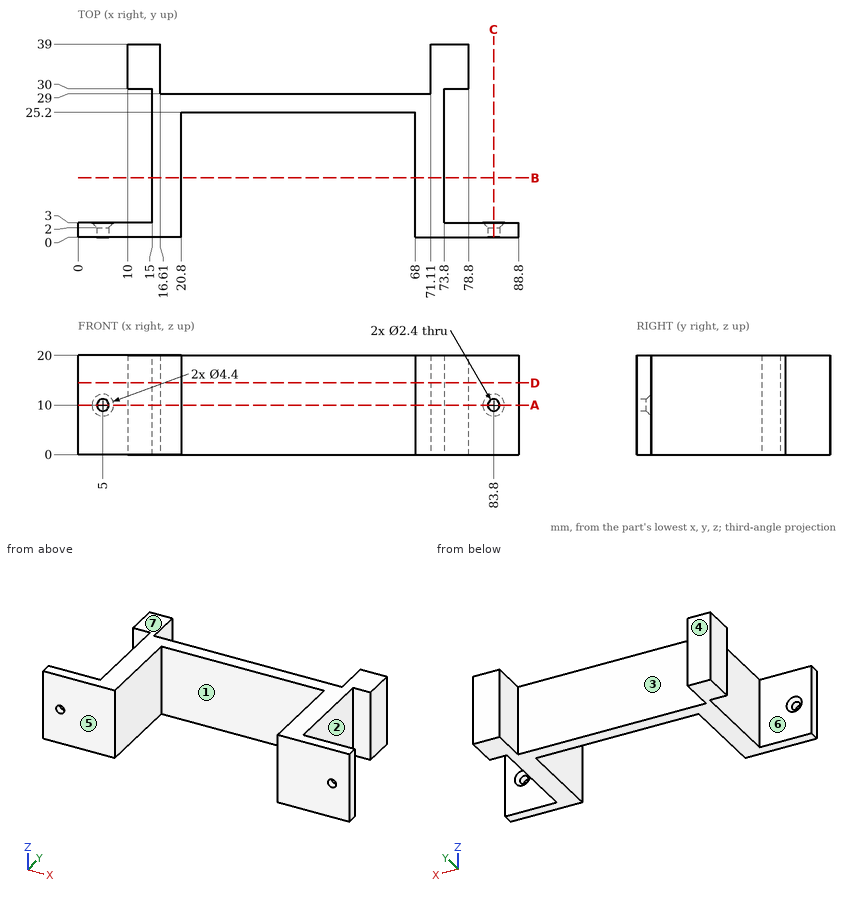
Design review of the part shown in the three views and the two pictorial views. Dimensions are in mm from the part's minimum x, y and z. A direction names the side the tool comes from. Give positions to 0.01 mm unless a question says otherwise; leave off trailing zeros. Write each loop counter-clockwise with the first axis right and the second up, starting at its lowest first coordinate (ties: lowest second). Pieces come first, ordered by that corner, then holes. Notation, with made-up numbers: M 36,45.25 L 76,45.25 A8 ccw 76,55.25 Z; hole C 39,12 d7. An arc over 180 degrees is marked long. Answer as CSV lines item,"result".
1. Draft analysis for pull direction Y (two halves, no side actions). For the marked faces 4, 5, 6 and 7, state which applies: +Y half, -Y half, draft (parallel to the pull), parting line (faces both ways), or undercut.
Findings:
face 4,"+Y half"
face 5,"-Y half"
face 6,"undercut"
face 7,"draft"
2. For the marked faces 1, 2 and 3, list the 3-axis set-ups (+Z, -Z, +X, -X, +Y, -Y) from which the entire face can be reached by the end or side of a thin tool; tool diameter is ignored.
Findings:
face 1,"+Z, -Z, -Y"
face 2,"+Z, -Z, +X"
face 3,"+Z, -Z, +Y"
3. Consider section B-B, the plane y = 12. Write out the cut boundary in (x, z), then the cut area to 3 significant figures.
Findings:
outline,"M 15,0 L 20.8,0 L 20.8,20 L 15,20 Z; M 68,0 L 73.8,0 L 73.8,20 L 68,20 Z"
area,"232 mm2"
4. Consider section C-C, the plane x = 83.8. Write out the cut boundary in (y, z), then the cut area to 3 significant figures.
Findings:
outline,"M 0,0 L 3,0 L 3,7.8 L 2,8.8 L 0,8.8 Z; M 0,11.2 L 2,11.2 L 3,12.2 L 3,20 L 0,20 Z"
area,"51.8 mm2"
5. Wall thickness on line 1 (X direction, y = 1.15, z = 10); line 2 (X direction, y = 15, z = 4.5); line 3 (Z direction, x = 5, y = 1.25): over which ranges is each line inside the solid? List them lowest first.
Findings:
line 1,"x = 0 to 3.8, 6.2 to 20.8, 68 to 82.6, 85 to 88.8"
line 2,"x = 15 to 20.8, 68 to 73.8"
line 3,"z = 0 to 8.8, 11.2 to 20"
6. Consider section A-A, the plane z = 10. Count the separate pieces of the cut face and the enclosed holes in it, then the cut area to 3 significant figures.
Findings:
separate pieces,"3"
enclosed holes,"0"
area,"722 mm2"
7. For pin 1 (10 mm diameter, centred on y = 10.5, z = 13, fed in from -X); pin 2 (1 mm diameter, centred on x = 15.5, z = 16.5, fed in from -Y); pin 3 (12 mm diameter, centred on y = 30.5, z = 12, fed in from +X); pin 4 (10 mm diameter, centred on y = 16, z = 12.5, fed in from +X), all flat-tipped, find the tip position at first contact; note any pin that passes through.
Findings:
pin 1,"stops at x = 15"
pin 2,"stops at y = 0"
pin 3,"stops at x = 78.8"
pin 4,"stops at x = 73.8"
8. Consider section D-D, the plane z = 14.5. Write out the cut boundary in (x, y).
Findings:
outline,"M 0,0 L 20.8,0 L 20.8,25.2 L 68,25.2 L 68,0 L 88.8,0 L 88.8,3 L 73.8,3 L 73.8,30 L 78.8,30 L 78.8,39 L 71.11,39 L 71.11,29 L 16.61,29 L 16.61,39 L 10,39 L 10,30 L 15,30 L 15,3 L 0,3 Z"
